from build123d import *

# Parameters (mm, degrees)
BOSS_EXTRUDE1_DEPTH = 14.5
SHELL1_T            = -2
SKETCH3_R           = 1.25
SKETCH3_W           = 25
SKETCH3_H           = 68.14690015
BOSS_EXTRUDE2_DEPTH = 1
CUT_EXTRUDE1_DEPTH  = 2


with BuildPart() as part:
    # Sketch1 → Boss-Extrude1 (new body, symmetric)
    with BuildSketch(Plane(origin=(0, 0, 0), x_dir=(0, 0, -1), z_dir=(1, 0, 0))):
        with BuildLine():
            Line((-36.124783736, -8), (36.124783736, -8))
            ThreePointArc((36.124783736, -8), (0, 37), (-36.124783736, -8))
        make_face()
    extrude(amount=BOSS_EXTRUDE1_DEPTH, both=True)

    # Shell1
    shell1_openings = [part.faces().sort_by_distance(p)[0] for p in [
        (0, -8, 0),
    ]]
    offset(amount=SHELL1_T, openings=shell1_openings)

    # Sketch3 → Boss-Extrude2 (add, symmetric)
    with BuildSketch(Plane.XZ.offset(8)):
        with BuildLine():
            Line((-9.5, 44.073450075), (17.5, 44.073450075))
            ThreePointArc((17.5, 44.073450075), (21.035533906, 42.608983981), (22.5, 39.073450075))
            Line((22.5, 39.073450075), (22.5, -39.073450075))
            ThreePointArc((22.5, -39.073450075), (21.035533906, -42.608983981), (17.5, -44.073450075))
            Line((17.5, -44.073450075), (-9.5, -44.073450075))
            Line((-9.5, -44.073450075), (-14.5, -44.073450075))
            Line((-14.5, -44.073450075), (-14.5, -39.073450075))
            Line((-14.5, -39.073450075), (-14.5, 39.073450075))
            Line((-14.5, 39.073450075), (-14.5, 44.073450075))
            Line((-14.5, 44.073450075), (-9.5, 44.073450075))
        make_face()
        with Locations((18.5, 40.073450075)):
            Circle(SKETCH3_R, mode=Mode.SUBTRACT)
        with Locations((-8.5, 40.073450075)):
            Circle(SKETCH3_R, mode=Mode.SUBTRACT)
        with Locations((18.5, -40.073450075)):
            Circle(SKETCH3_R, mode=Mode.SUBTRACT)
        with Locations((-8.5, -40.073450075)):
            Circle(SKETCH3_R, mode=Mode.SUBTRACT)
        Rectangle(SKETCH3_W, SKETCH3_H, mode=Mode.SUBTRACT)
    extrude(amount=BOSS_EXTRUDE2_DEPTH, both=True)

    # Sketch4 → Cut-Extrude1 (cut)
    with BuildSketch(Plane(origin=(-12.5, 0, 0), x_dir=(0, 0, -1), z_dir=(1, 0, 0))):
        with BuildLine():
            Line((-44.073450075, -7), (-36.331804249, -7))
            ThreePointArc((-36.331804249, -7), (0, 37), (36.331804249, -7))
            Line((36.331804249, -7), (44.073450075, -7))
            Line((44.073450075, -7), (44.073450075, -9))
            Line((44.073450075, -9), (-44.073450075, -9))
            Line((-44.073450075, -9), (-44.073450075, -7))
        make_face()
    extrude(amount=-CUT_EXTRUDE1_DEPTH, mode=Mode.SUBTRACT)


solid = part.part
Could you check a few things on this model? Use its own coordinates, in mm. A direction names the side the tool comes from. Give positions to 0.01 mm unless a question says otherwise; leave off trailing zeros. Write each loop counter-clockwise with the first axis right and the second up, starting at its lowest first coordinate (ties: lowest second). Pieces come first, ordered by that corner, then holes. Notation, with made-up numbers: (56, -22.75) -> (79, -22.75) arc R18 ccw to (79, -12.75) -> close; hole circle Ø5 at (37, 86.25). An arc over 180 degrees is marked (long way). Answer as a JSON object with one key per item and string values.
Q1. Please list where these lines run through material, in increasing order: L1, parallel to Z at x = 18, y = -8; L2, parallel to Z at x = 3, y = 0; L3, parallel to X at y = -3, z = -5.
Taken from the geometry:
{"L1": "z = -44.05 to -41.22, -38.93 to 38.93, 41.22 to 44.05", "L2": "z = -37 to -35, 35 to 37", "L3": "x = 12.5 to 14.5"}
Q2. Suppose I cut it at B-B on x = 18.5. Write out the boundary of the cut face in (y, z).
Taken from the geometry:
{"outline": "(-9, -43.97) -> (-7, -43.97) -> (-7, -41.32) -> (-9, -41.32) -> close; (-9, -38.82) -> (-7, -38.82) -> (-7, 38.82) -> (-9, 38.82) -> close; (-9, 41.32) -> (-7, 41.32) -> (-7, 43.97) -> (-9, 43.97) -> close"}
Q3. Suppose I cut it at D-D on x = 1. Write out the boundary of the cut face in (y, z).
Taken from the geometry:
{"outline": "(-9, -44.07) -> (-7, -44.07) -> (-7, -36.33) arc R37 ccw (long way) to (-7, 36.33) -> (-7, 44.07) -> (-9, 44.07) -> (-9, 34.07) -> (-7, 34.07) -> (-7, 34.29) arc R35 cw (long way) to (-7, -34.29) -> (-7, -34.07) -> (-9, -34.07) -> close"}
Q4. Which directions (+Z, -Z, +X, -X, +Y, -Y) give clear straight access to the entire face, cutting with the end or side of a thin tool? Please do faces 1 (the flat face through (0, -8, 34.073)), 2 (the flat face through (22.5, -8, 1)), 3 (the cylindrical face through (0.18, 34.99, -0.87)).
Taken from the geometry:
{"face 1": "-X, -Y", "face 2": "+Z, -Z, +X, +Y, -Y", "face 3": "-X"}
Q5. Suppose I cut it at C-C on z = 0. Write out the boundary of the cut face in (x, y).
Taken from the geometry:
{"outline": "(-12.5, 35) -> (12.5, 35) -> (12.5, -9) -> (22.5, -9) -> (22.5, -7) -> (14.5, -7) -> (14.5, 37) -> (-12.5, 37) -> close"}
Q6. We'd pull the mould along Z, two halves only. Please class faces 4 (the cylindrical face through (20.996, -8.014, 42.648)), 5 (the flat face through (14.5, 10, 1)), 6 (the cylindrical face through (-9.49, -7.99, 39.31)): released by +Z, released by -Z, zero draft, split by the parting line, or undercut.
Taken from the geometry:
{"face 4": "released by +Z", "face 5": "zero draft", "face 6": "undercut"}
Q7. Suppose I cut it at A-A on y = 0. Write out the boundary of the cut face in (x, z), then the cut area to 3 significant figures.
Taken from the geometry:
{"outline": "(-12.5, -37) -> (14.5, -37) -> (14.5, 37) -> (-12.5, 37) -> (-12.5, 35) -> (12.5, 35) -> (12.5, -35) -> (-12.5, -35) -> close", "area": "248 mm²"}
Q8. Will these pins go through, and if not, where does the flat tip stop? pin 1 Ø4 at (x, y) = (-3.5, 16) entering from +Z; pin 2 Ø6 at (x, y) = (6.5, 25) entering from -Z; pin 3 Ø12 at (y, z) = (1, 14.5) entering from +X.
Taken from the geometry:
{"pin 1": "stops at z = 34.25", "pin 2": "stops at z = -29.75", "pin 3": "stops at x = 14.5"}
